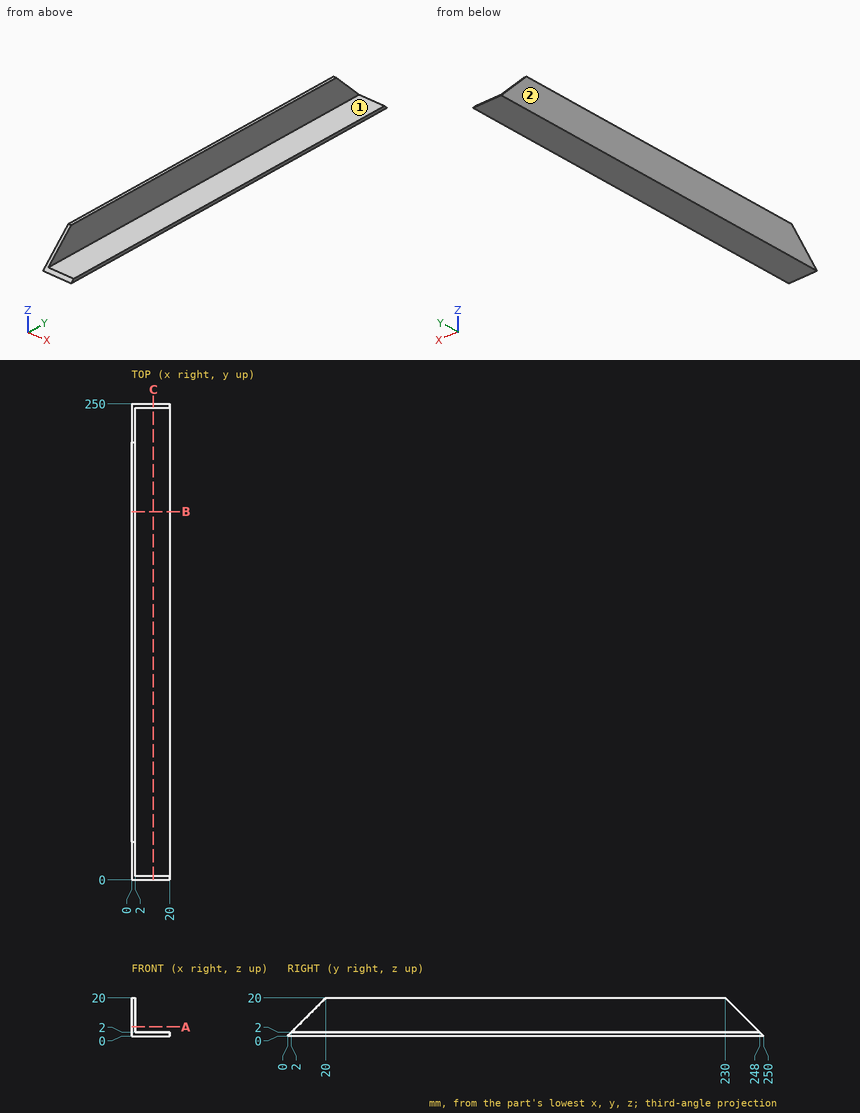
Could you check a few things on this drawing? It's one solid part, dimensions in mm from its lowest x, y, z. A direction names the side the tool comes from. Give positions to 0.01 mm unless a question says otherwise; leave off trailing zeros. Order: outer loops, then holes, each group sorted by start corner. A loop starts at its lowest first (then second) coordinate and runs counter-clockwise, first axis right, second up. Notation, with made-up numbers: (89.25, 71) - (145.25, 71) arc R20 ccw to (145.25, 104) - close; hole circle Ø4 at (-3, 76). An arc over 180 degrees is marked (long way). One line per question, with ' | ' between items. Start each with the question number.
Item 1: I want a section at A-A on z = 4.75. Write out the boundary of the cut face in (x, y), then the cut area to 3 significant figures.
Item 2: I want a section at C-C on x = 11.5. Write out the boundary of the cut face in (y, z), then the cut area to 3 significant figures.
Item 3: For the marked faces 1 and 2, which set-ups out of +Z, -Z, +X, -X, +Y, -Y let a thin tool reach every point of the face, with its end or its side?
Item 4: I need wall thicknesses on probe 1 along Z at (x, y) = (3, 175); probe 2 along Y at (x, z) = (14, 1.75). Which ranges of each line are inside material? Lowest first, please. Write a range as [from, to].
Item 5: I'm going to push flat-ended pins straight in: pin 1 Ø8 at (y, z) = (198, 11) entering from -X; pin 2 Ø5 at (x, z) = (3.5, 6) entering from -Y; pin 3 Ø10 at (x, z) = (3, 14.5) entering from -Y; pin 4 Ø4 at (x, y) = (14, 38.5) entering from +Z. Where does each tip first touch, or does it pass through?
Item 6: I want a section at B-B on y = 193.5. Write out the boundary of the cut face in (x, z), then the cut area to 3 significant figures.
Verdict:
1) outline: (0, 4.75) - (2, 4.75) - (2, 245.25) - (0, 245.25) - close | area: 481 mm^2
2) outline: (0, 0) - (250, 0) - (248, 2) - (2, 2) - close | area: 496 mm^2
3) face 1: +Z, +X, +Y, -Y | face 2: +Z, -Z, -X, +Y, -Y
4) probe 1: [0, 2] | probe 2: [1.75, 248.25]
5) pin 1: x = 0 | pin 2: y = 4 | pin 3: y = 9.6 | pin 4: z = 2
6) outline: (0, 0) - (20, 0) - (20, 2) - (2, 2) - (2, 20) - (0, 20) - close | area: 76.0 mm^2
